The listing builds one solid part. Answer for the finished solid, in the listing's coordinates (mm). A direction names the side the tool comes from. Round coordinates to 2 decimals unless told otherwise and drop trailing zeros. Loops run counter-clockwise (first coordinate to the right, second up) from the corner with the lowest first, then second, coordinate; pieces in that order, holes last. Notation, with made-up numbers: (88.5, -8.75) -> (122.5, -8.75) arc R37 cw to (122.5, 27.25) -> close; hole circle Ø6 at (26, -26.75). An arc over 180 degrees is marked (long way). Write each question's results on one line, items separated by ' | '. Start each with the question number.
from build123d import *

# Parameters (mm, degrees)
ENLEV_MAT_EXTRU1_DEPTH = 2
ESQUISSE3_W            = 2
ESQUISSE3_H            = 20
CHANFREIN1_SIZE        = 0.4


with BuildPart() as part:
    # Esquisse1 → Base-Révolution (revolve)
    with BuildSketch(Plane(origin=(0, 0, 0), x_dir=(1, 0, 0), z_dir=(0, 1, 0)), mode=Mode.PRIVATE) as base_r_volution_sk:
        with BuildLine():
            Line((0, 0), (3.5, 0))
            Line((3.5, 0), (3.5, 3.6))
            ThreePointArc((3.5, 3.6), (3.382842712, 3.882842712), (3.1, 4))
            Line((3.1, 4), (0, 4))
            Line((0, 4), (0, 0))
        make_face()
    revolve(base_r_volution_sk.sketch.rotate(Axis((0, 0, 0), (0, 0, -1)), 180), axis=Axis((0, 0, 0), (0, 0, -1)))

    # Esquisse2 → enlev-mat-Extru1 (cut)
    with BuildSketch(Plane.XY.offset(-4)):
        Polygon((1.5, -0.866025404), (1.5, 0.866025404), (0, 1.732050808), (-1.5, 0.866025404), (-1.5, -0.866025404), (0, -1.732050808), align=None)
    extrude(amount=ENLEV_MAT_EXTRU1_DEPTH, mode=Mode.SUBTRACT)

    # Esquisse3 → Boss.-Révol.1 (revolve)
    with BuildSketch(Plane(origin=(0, 0, 0), x_dir=(1, 0, 0), z_dir=(0, 1, 0))):
        with Locations((1, -10)):
            Rectangle(ESQUISSE3_W, ESQUISSE3_H)
    revolve(axis=Axis((0, 0, 0), (0, 0, 1)))

    # Chanfrein1
    chanfrein1_edges = [part.edges().sort_by_distance(p)[0] for p in [
        (-2, 0, 20),
    ]]
    chamfer(chanfrein1_edges, length=CHANFREIN1_SIZE)


solid = part.part
Item 1: The part is cut by section B-B, the plane z = -0.75. Give the vertices of the cut face in (x, y), plus the area to 3 significant figures.
Item 2: Each of these flat-tipped pins is pushed along its axis until it touches: pin 1 Ø4 at (x, z) = (-1, 1) entering from -Y; pin 2 Ø0.5 at (y, z) = (0.5, -2.5) entering from +X; pin 3 Ø4 at (x, z) = (-0.5, 11) entering from +Y; pin 4 Ø1 at (y, z) = (-0.5, 11.5) entering from -X. Where does it stop, or does it pass through?
Item 3: The part is cut by section A-A, the plane y = 0. Give the vertices of the cut face in (x, z).
Item 4: For faces 1 (the cylindrical face through (0, -2, 10)), 2 (the flat face through (0, 0, 20)), 3 (the flat face through (0.74, -1.305, -3.014)), determine the directions among +Z, -Z, +X, -X, +Y, -Y from which every point of the face is accessible in a straight line to the end or side of a thin tool.
Item 5: Straight lines are drawn through the part: L1, parallel to Z at x = 2.5, y = 0.75; L2, parallel to X at y = -1, z = 17.25. For each, find the intervals that lie inside material, in ascending order. Write a range as [from, to].
Item 6: Determine the mould class of faces 4 (the flat face through (-1.3, -1.3, -4)), 5 (the cylindrical face through (-3.233, -1.341, -1.825)), 6 (the flat face through (-0.76, -1.293, -3.014)) for opening direction X: +X half, -X half, draft (parallel to the pull), parting line (faces both ways), or undercut.
Item 7: The part is cut by section C-C, the plane z = 17.25. Give the vertices of the cut face in (x, y), plus the area to 3 significant figures.
Report:
1) outline: circle Ø7 at (0, 0) | area: 38.5 mm2
2) pin 1: stops at y = -3.5 | pin 2: stops at x = 3.49 | pin 3: stops at y = 2 | pin 4: stops at x = -2
3) outline: (-3.5, -3.6) arc R0.4 ccw to (-3.1, -4) -> (-1.5, -4) -> (-1.5, -2) -> (1.5, -2) -> (1.5, -4) -> (3.1, -4) arc R0.4 ccw to (3.5, -3.6) -> (3.5, 0) -> (2, 0) -> (2, 19.6) -> (1.6, 20) -> (-1.6, 20) -> (-2, 19.6) -> (-2, 0) -> (-3.5, 0) -> close
4) face 1: +Z | face 2: +Z, +X, -X, +Y, -Y | face 3: -Z
5) L1: z = [-4, 0] | L2: x = [-1.73, 1.73]
6) face 4: draft | face 5: parting line | face 6: undercut
7) outline: circle Ø4 at (0, 0) | area: 12.6 mm2
